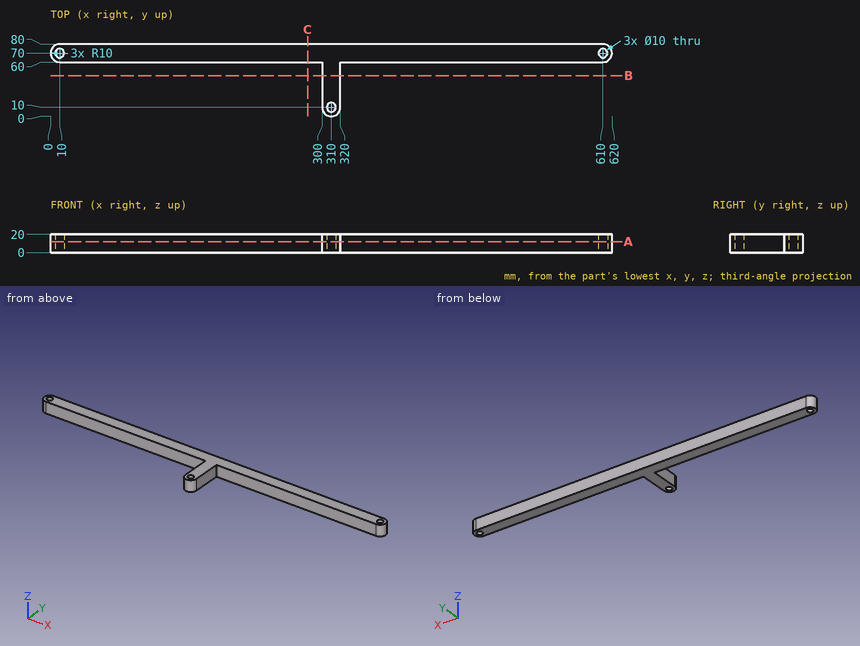
The drawing under review shows one solid part. Ordinate dimensions are in mm from its lowest x, y, z. Give positions to 0.01 mm unless a question says otherwise; leave off trailing zeros. Write each loop counter-clockwise with the first axis right and the second up, starting at its lowest first coordinate (ties: lowest second). Pieces come first, ordered by that corner, then holes.
1. Wall thickness on L1, parallel to Y at x = 310, z = 9.25; L2, parallel to Y at x = 610, z = 14.5; L3, parallel to X at y = 68, z = 1.25: over which ranges is each line inside the solid? List them lowest first.
2. Add section A-A, the plane z = 12. Write out the cut boundary in (x, y), plus the area to 3 significant figures.
3. Add section B-B, the plane y = 45. Write out the cut boundary in (x, z), plus the area to 3 significant figures.
4. Add section C-C, the plane x = 284. Write out the cut boundary in (y, z), plus the area to 3 significant figures.
5. For P1, Ø13, axis at x = 610, y = 70, coming from the -Z side; P2, Ø10, axis at y = 13.5, z = 15.5, coming from the -X side; P3, Ø2, axis at x = 316.5, z = 14, coming from the -Y side; P4, Ø2, axis at y = 23.5, z = 13, coming from the +X side, all flat-tipped, find the tip position at first contact; note any pin that passes through.
Worked answers:
1. L1: y = 0 to 5, 15 to 80
1. L2: y = 60 to 65, 75 to 80
1. L3: x = 0.2 to 5.42, 14.58 to 605.42, 614.58 to 619.8
2. outline: (10, 60) - (300, 60) - (300, 10) arc R10 ccw to (320, 10) - (320, 60) - (610, 60) arc R10 ccw to (610, 80) - (10, 80) arc R10 ccw to start; hole circle Ø10 at (10, 70); hole circle Ø10 at (310, 10); hole circle Ø10 at (610, 70)
2. area: 13,200 mm2
3. outline: (300, 0) - (320, 0) - (320, 20) - (300, 20) - close
3. area: 400 mm2
4. outline: (60, 0) - (80, 0) - (80, 20) - (60, 20) - close
4. area: 400 mm2
5. P1: stops at z = 0
5. P2: stops at x = 300
5. P3: stops at y = 1.65
5. P4: stops at x = 320
